Autodesk Inventor part; units mm, degrees
ref_plane "YZ Plane" through (0, 0, 0) normal (1, 0, 0) x (0, 1, 0)
ref_plane "XZ Plane" through (0, 0, 0) normal (0, 1, 0) x (-1, 0, 0)
ref_plane "XY Plane" through (0, 0, 0) normal (0, 0, 1) x (1, 0, 0)
sketch "Sketch1" plane through (0, 0, 0) normal (0, 1, 0) x (-1, 0, 0)
  circle A0 centre (0, 0) radius 190.5
  circle A1 centre (0, 0) radius 60.325
  dimension "d0" = 381
  dimension "d1" = 120.65
extrude "Extrusion1" add sketch "Sketch1" along normal blind 12.7
sketch "Sketch2" plane through (0, 12.7, 0) normal (0, 1, 0) x (1, 0, 0)
  line L0 (-142.875, 63.5) -> (-136.525, 63.5)
  line L1 (-136.525, 63.5) -> (-136.525, 50.8)
  line L2 (-136.525, 50.8) -> (-142.875, 50.8)
  line L3 (-142.875, 50.8) -> (-142.875, 63.5)
  line L4 (-136.525, 50.8) -> (-136.525, -50.8) construction
  line L5 (-111.125, 50.8) -> (-212.725, 50.8) construction
  line L6 (-136.525, -50.8) -> (-142.875, -50.8)
  line L7 (-142.875, -50.8) -> (-142.875, -38.1)
  line L8 (-142.875, -38.1) -> (-136.525, -38.1)
  line L9 (-136.525, -38.1) -> (-136.525, -50.8)
  line L10 (-136.525, 0) -> (-60.325, 0) construction
  line L11 (-136.525, 0) -> (-60.325, 0) construction
  circle A0 centre (0, 0) radius 85.725 construction
  line L12 (0, 0) -> (-85.725, 0) construction
  dimension "d4" = 6.35
  dimension "d5" = 12.7
  dimension "d6" = 101.6
  dimension "d7" = 90
  dimension "d8" = 6.35
  dimension "d9" = 12.7
  dimension "d10" = 76.2
  dimension "d11" = 0
extrude "Extrusion2" cut sketch "Sketch2" against normal through all
sketch "Sketch3" plane through (0, 12.7, 0) normal (0, 1, 0) x (1, 0, 0)
  circle A0 centre (0, 0) radius 157.48 construction
  circle A1 centre (-157.48, 0) radius 3.9687
  circle A2 centre (-78.74, -136.3817) radius 3.9687
  circle A3 centre (78.74, -136.3817) radius 3.9687
  circle A4 centre (157.48, 0) radius 3.9687
  circle A5 centre (78.74, 136.3817) radius 3.9687
  circle A6 centre (-78.74, 136.3817) radius 3.9687
  dimension "d16" = 314.96
  dimension "d17" = 7.9375
  dimension "d18" = 360
extrude "Extrusion3" cut sketch "Sketch3" against normal through all
sketch "Sketch4" plane through (0, 12.7, 0) normal (0, 1, 0) x (1, 0, 0)
  line L0 (0, 0) -> (0, -177.8) construction
  line L1 (0, 0) -> (177.8, 0) construction
  circle A0 centre (0, -177.8) radius 3.81
  circle A1 centre (153.9793, -88.9) radius 3.81
  circle A2 centre (153.9793, 88.9) radius 3.81
  circle A3 centre (0, 177.8) radius 3.81
  circle A4 centre (-153.9793, 88.9) radius 3.81
  circle A5 centre (-153.9793, -88.9) radius 3.81
  dimension "d21" = 177.8
  dimension "d22" = 90
  dimension "d23" = 7.62
  dimension "d26" = 360
extrude "Extrusion4" cut sketch "Sketch4" against normal through all
sketch "Sketch5" plane through (0, 12.7, 0) normal (0, 1, 0) x (1, 0, 0)
  circle A0 centre (-157.48, 0) radius 3.9687
  circle A1 centre (-157.48, 0) radius 12.7
  point P0 (0, 0)
  dimension "d30" = 25.4
extrude "Extrusion5" cut sketch "Sketch5" against normal through all
equation "\"d4\" = d8"
properties part number "Turntable Top" material "PVC-Piping"
Design review of the part built by this model. Coordinates are the model's own, in mm. A direction names the side the tool comes from. Coordinates: 2 decimals unless noted, no trailing zeros. Loops run counter-clockwise (first coordinate to the right, second up) from the corner with the lowest first, then second, coordinate; pieces in that order, holes last.
Item 1: Clearance check with flat-ended pins moving along their axes: pin 1 (5 mm diameter, centred on x = -140.5, y = 5, fed in from +Z) (3 decimals); pin 2 (3 mm diameter, centred on x = -138.5, y = 8.5, fed in from +Z); pin 3 (4.5 mm diameter, centred on x = 153.98, z = 88.9, fed in from +Y); pin 4 (7 mm diameter, centred on x = -138.5, y = 4, fed in from -Z). State where each tip first meets the part, or that it passes through.
Completed:
pin 1: stops at z = 131.325
pin 2: stops at z = 132.37
pin 3: passes through
pin 4: stops at z = -134.41
Item 2: Wall thickness on L1, parallel to X at y = 8.75, z = -88.9; L2, parallel to Z at x = 0, y = 9.75 (3 decimals); L3, parallel to X at y = 6.75, z = 8: over which ranges is each line inside the solid? List them lowest first.
Completed:
L1: x = -168.48 to -157.79, -150.17 to 150.17, 157.79 to 168.48
L2: z = -190.5 to -181.61, -173.99 to -60.325, 60.325 to 173.99, 181.61 to 190.5
L3: x = -190.33 to -167.34, -147.62 to -59.79, 59.79 to 190.33
Item 3: Add section B-B (z = 19.5). Write out the cut boundary in (x, y).
Completed:
outline: (-189.5, 0) - (-57.09, 0) - (-57.09, 12.7) - (-189.5, 12.7) - close; (57.09, 0) - (189.5, 0) - (189.5, 12.7) - (57.09, 12.7) - close
Item 4: For faces 1 (the flat face through (-142.875, 6, 45)), 2 (the flat face through (45, 12.7, 45)), list the 3-axis set-ups (+Z, -Z, +X, -X, +Y, -Y) from which the entire face can be reached by the end or side of a thin tool; tool diameter is ignored.
Completed:
face 1: +Y, -Y
face 2: +Z, -Z, +X, -X, +Y
Item 5: Draft analysis for pull direction Z (two halves, no side actions). For faces 3 (the flat face through (-136.525, 6, 44)), 4 (the cylindrical face through (151.17, 6.26, 115.92)), 5 (the flat face through (45, 0, 45)), 6 (the cylindrical face through (-170.168, 6.439, -0.558)), state which applies: pulls with the +Z half, pulls with the -Z half, needs draft (parallel to the pull), parting line crosses it, or undercut.
Completed:
face 3: undercut
face 4: parting line crosses it
face 5: needs draft
face 6: undercut
Item 6: Add section D-D (z = 126). Write out the cut boundary in (x, y), and give its area (3 significant figures).
Completed:
outline: (-142.88, 0) - (142.88, 0) - (142.88, 12.7) - (-142.88, 12.7) - close
area: 3,630 mm2
Item 7: Add section A-A (x = -34). Write out the cut boundary in (y, z), and give its area (3 significant figures).
Completed:
outline: (0, -187.44) - (12.7, -187.44) - (12.7, -49.83) - (0, -49.83) - close; (0, 49.83) - (12.7, 49.83) - (12.7, 187.44) - (0, 187.44) - close
area: 3,500 mm2
Item 8: Add section C-C (z = -159). Write out the cut boundary in (x, y).
Completed:
outline: (-104.92, 0) - (104.92, 0) - (104.92, 12.7) - (-104.92, 12.7) - close
